```python
from build123d import *

# Parameters (mm, degrees)
SKIZZE2_R                       = 95
SKIZZE2_R_2                     = 75
AUFSATZ_LINEAR_AUSTRAGEN1_DEPTH = 20
SKIZZE3_W                       = 25
SKIZZE3_H                       = 25
VERRUNDUNG3_R                   = 2


with BuildPart() as part:
    # Skizze2 → Aufsatz-Linear austragen1 (new body)
    with BuildSketch(Plane.XY):
        Circle(SKIZZE2_R)
        Circle(SKIZZE2_R_2, mode=Mode.SUBTRACT)
    extrude(amount=AUFSATZ_LINEAR_AUSTRAGEN1_DEPTH)

    # Skizze3 → Rotation1 (revolve)
    with BuildSketch(Plane(origin=(0, 0, 0), x_dir=(1, 0, 0), z_dir=(0, 1, 0))):
        with Locations((87.5, -32.5)):
            Rectangle(SKIZZE3_W, SKIZZE3_H)
    revolve(axis=Axis((0, 0, 20), (0, 0, -1)))

    # Verrundung3
    verrundung3_edges = [part.edges().sort_by_distance(p)[0] for p in [
        (-100, 0, 20),
        (-95, 0, 20),
    ]]
    fillet(verrundung3_edges, radius=VERRUNDUNG3_R)


solid = part.part
```
Geometry check sheet. Reference: the model listing, model coordinates, mm. A direction names the side the tool comes from. Give positions to 0.01 mm unless a question says otherwise; leave off trailing zeros. Order: outer loops, then holes, each group sorted by start corner. A loop starts at its lowest first (then second) coordinate and runs counter-clockwise, first axis right, second up.
1. Gauge pin test, flat ends, axial feed: pin 1 Ø10 at (x, z) = (-78, 13.5) entering from +Y; pin 2 Ø1 at (x, z) = (-23, 24.5) entering from -Y; pin 3 Ø6 at (y, z) = (-61.5, 28) entering from -X. Record the tip position at first contact, or that the pin passes through.
2. Section check D-D, the plane z = 4.5. Enter the section's corners in (x, y), and give its area (3 significant figures).
3. Release check for a two-part mould opening along Y. For faces 1 (the face through (70, 29, 0)), 2 (the face through (-9.764, -74.362, 22.185)), 3 (the face through (95.38, -30.04, 33.34)) record: pulls with the +Y half, pulls with the -Y half, needs draft (parallel to the pull), parting line crosses it, or undercut.
4. Section check C-C, the plane z = 27.5. Enter the section's corners in (x, y).
5. Access from +Z, -Z, +X, -X, +Y, -Y to the whole of each face (thin tool, end or side, straight path). Record for faces 4 (the face through (-14, -75, 45)), 5 (the face through (95, -22, 20)).
6. Section check A-A, the plane y = 0. Enter the section's corners in (x, z).
7. Thickness scan on L1, parallel to X at y = 0, z = 30.5; L2, parallel to X at y = 47, z = 24. Record the ranges inside material, lowest first.
Values follow:
1. pin 1: stops at y = 60.79
1. pin 2: stops at y = -97.44
1. pin 3: stops at x = -81.1
2. outline: circle Ø190 at (0, 0); hole circle Ø150 at (0, 0)
2. area: 10,700 mm2
3. face 1: needs draft
3. face 2: undercut
3. face 3: parting line crosses it
4. outline: circle Ø200 at (0, 0); hole circle Ø150 at (0, 0)
5. face 4: +Z, +X, -X, +Y, -Y
5. face 5: -Z
6. outline: (-100, 22) arc R2 ccw to (-98, 20) - (-97, 20) arc R2 cw to (-95, 18) - (-95, 0) - (-75, 0) - (-75, 45) - (-100, 45) - close; (75, 0) - (95, 0) - (95, 18) arc R2 cw to (97, 20) - (98, 20) arc R2 ccw to (100, 22) - (100, 45) - (75, 45) - close
7. L1: x = -100 to -75, 75 to 100
7. L2: x = -88.27 to -58.45, 58.45 to 88.27
